Read the model definition and answer for the solid it produces. Units are mm, in the model's axes. Face numbers are marked on the shaded views. Coordinates: 2 decimals unless noted, no trailing zeros. Loops run counter-clockwise (first coordinate to the right, second up) from the corner with the lowest first, then second, coordinate; pieces in that order, holes last. Notation, with made-up numbers: (-16.75, 53.5) -> (20.25, 53.5) arc R25 cw to (20.25, 89.5) -> close; hole circle Ø1 at (32.25, 66). An arc over 180 degrees is marked (long way). Answer as a JSON object with one key per item and string values. Group by question number.
1) Section C-C, the plane y = 28.5 is taken. Give the vertices of the cut face in (x, z).
2) Consider probe 1 along Y at (x, z) = (-7, 5.25); probe 2 along Z at (x, y) = (0, 2); probe 3 along Z at (x, y) = (-52, 55.5). Determine where each line is inside the solid, lowest interval first. Write a range as [from, to].
3) Section A-A, the plane z = -11.5 is taken. Give the vertices of the cut face in (x, y), plus the area to 3 significant figures.
4) Flat-ended cylindrical pins translate along their axes: P1, Ø8.5, axis at x = -14, z = 3, coming from the +Y side; P2, Ø1, axis at x = -11, z = 11, coming from the -Y side; P3, Ø16, axis at y = 40.5, z = 0, coming from the +X side. Find the tip coordinate at first contact, or state that the pin passes through.
5) Section B-B, the plane x = -36 is taken. Give the vertices of the cut face in (y, z).
6) Section D-D, the plane z = 0 is taken. Count the separate pieces of the cut face and the enclosed holes in it, plus the area to 3 significant figures.
7) Determine the mould class of the marked faces 1, 2, 3 and 4 for opening direction Y: released by +Y, released by -Y, zero draft, split by the parting line, or undercut.
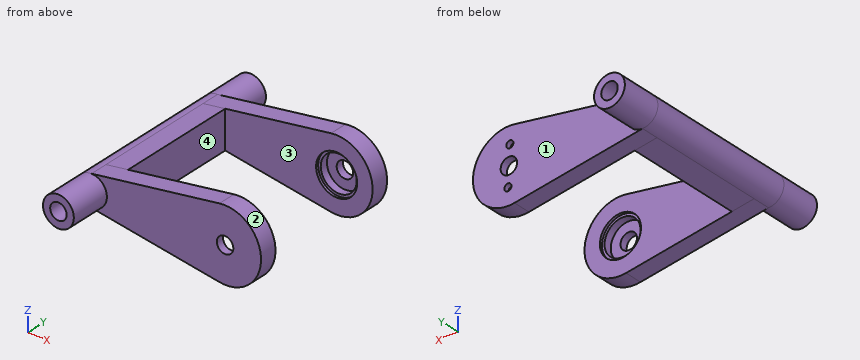
from build123d import *

# Parameters (mm, degrees)
SKETCH1_R               = 3.2
BOSS_EXTRUDE1_DEPTH     = 7
SKETCH2_R               = 3.2
BOSS_EXTRUDE2_DEPTH     = 47
BOSS_EXTRUDE3_OUTLINE_R = 3.2
BOSS_EXTRUDE3_DEPTH     = 7
CUT_EXTRUDE1_DEPTH      = 86.32877599
CUT_EXTRUDE1_DEPTH_BACK = 86.32877599
SKETCH5_R               = 3.2
SKETCH6_R               = 1.395
CUT_EXTRUDE2_DEPTH      = 2
SKETCH7_R               = 7
CUT_EXTRUDE3_DEPTH      = 4
SKETCH8_R               = 8
CUT_EXTRUDE4_DEPTH      = 1
CUT_EXTRUDE5_START      = -4
SKETCH9_R               = 7
CUT_EXTRUDE5_DEPTH      = 4
CUT_EXTRUDE6_START      = -1
SKETCH10_R              = 8
CUT_EXTRUDE6_DEPTH      = 1
SKETCH11_R              = 6
SKETCH11_R_2            = 3.2
BOSS_EXTRUDE4_DEPTH     = 16
BOSS_EXTRUDE5_START     = 16
SKETCH12_R              = 6
SKETCH12_R_2            = 3.2
BOSS_EXTRUDE5_DEPTH     = 16


# Read off the part's stored shape, not the designer's step: Boss-Extrude3
with BuildPart() as part:
    # Sketch1 → Boss-Extrude1 (new body)
    with BuildSketch(Plane(origin=(0, 0, 0), x_dir=(1, 0, 0), z_dir=(0, 1, 0))):
        with BuildLine():
            ThreePointArc((-52, 6), (-58, 0), (-52, -6))
            Line((-52, -6), (-2.173431493, -13.830264184))
            ThreePointArc((-2.173431493, -13.830264184), (14.000000424, -1.65e-07), (-2.173431166, 13.830264236))
            Line((-2.173431166, 13.830264236), (-52, 6))
        make_face()
        with Locations(Location((-52, 0, 0), (0, 0, 270))):
            Circle(SKETCH1_R, mode=Mode.SUBTRACT)
    extrude(amount=BOSS_EXTRUDE1_DEPTH)

    # Sketch2 → Boss-Extrude2 (add)
    # profile 1 of 2: a face of its own
    with BuildSketch(Plane(origin=(0, 7, 0), x_dir=(1, 0, 0), z_dir=(0, 1, 0))):
        with BuildLine():
            ThreePointArc((-46, 0), (-47.757359313, 4.242640687), (-52, 6))
            ThreePointArc((-52, 6), (-58, 0), (-52, -6))
            ThreePointArc((-52, -6), (-47.757359313, -4.242640687), (-46, 0))
        make_face()
        with Locations(Location((-52, 0, 0), (0, 0, 270))):
            Circle(SKETCH2_R, mode=Mode.SUBTRACT)
    # profile 2 of 2: a face of its own
    with BuildSketch(Plane(origin=(0, 7, 0), x_dir=(1, 0, 0), z_dir=(0, 1, 0))):
        with BuildLine():
            Line((-43.357698304, -7.358140997), (-43.357698304, 7.358140997))
            Line((-43.357698304, 7.358140997), (-52, 6))
            ThreePointArc((-52, 6), (-47.757359313, 4.242640687), (-46, 0))
            ThreePointArc((-46, 0), (-47.757359313, -4.242640687), (-52, -6))
            Line((-52, -6), (-43.357698304, -7.358140997))
        make_face()
    extrude(amount=BOSS_EXTRUDE2_DEPTH)

    # Boss-Extrude3 outline → Boss-Extrude3 (add)
    with BuildSketch(Plane(origin=(0, 54, 0), x_dir=(1, 0, 0), z_dir=(0, 1, 0))):
        with BuildLine():
            ThreePointArc((-2.17343128, -13.830264218), (14.000000424, -1.07e-07), (-2.173431068, 13.830264251))
            Line((-2.173431068, 13.830264251), (-52, 6))
            ThreePointArc((-52, 6), (-58, 0), (-52, -6))
            Line((-52, -6), (-2.17343128, -13.830264218))
        make_face()
        with Locations((-52, 0)):
            Circle(BOSS_EXTRUDE3_OUTLINE_R, mode=Mode.SUBTRACT)
    extrude(amount=BOSS_EXTRUDE3_DEPTH)

    # Sketch5 → Cut-Extrude1 (cut, two sides: drawn at the far end of the back side and taken through both)
    with BuildSketch(Plane(origin=(0, 61, 0), x_dir=(1, 0, 0), z_dir=(0, 1, 0)).offset(-CUT_EXTRUDE1_DEPTH_BACK)):
        with Locations(Location((0, 0, 0), (0, 0, 270))):
            Circle(SKETCH5_R)
    extrude(amount=CUT_EXTRUDE1_DEPTH + CUT_EXTRUDE1_DEPTH_BACK, mode=Mode.SUBTRACT)

    # Sketch6 → Cut-Extrude2 (cut)
    with BuildSketch(Plane(origin=(0, 61, 0), x_dir=(1, 0, 0), z_dir=(0, 1, 0))):
        with Locations(Location((-0.370638007, -7.432964974, 0), (0, 0, 270))):
            Circle(SKETCH6_R)
        with Locations(Location((0.370638007, 7.432964974, 0), (0, 0, 270))):
            Circle(SKETCH6_R)
    extrude(amount=-CUT_EXTRUDE2_DEPTH, mode=Mode.SUBTRACT)

    # Sketch7 → Cut-Extrude3 (cut)
    with BuildSketch(Plane.XZ.offset(-54)):
        with Locations(Location((0, 0, 0), (0, 0, 270))):
            Circle(SKETCH7_R)
    extrude(amount=-CUT_EXTRUDE3_DEPTH, mode=Mode.SUBTRACT)

    # Sketch8 → Cut-Extrude4 (cut)
    with BuildSketch(Plane.XZ.offset(-54)):
        with Locations(Location((0, 0, 0), (0, 0, 270))):
            Circle(SKETCH8_R)
    extrude(amount=-CUT_EXTRUDE4_DEPTH, mode=Mode.SUBTRACT)

    # Sketch9 → Cut-Extrude5 (cut)
    with BuildSketch(Plane(origin=(0, 7, 0), x_dir=(1, 0, 0), z_dir=(0, 1, 0)).offset(CUT_EXTRUDE5_START)):
        with Locations(Location((0, 0, 0), (0, 0, 90))):
            Circle(SKETCH9_R)
    extrude(amount=CUT_EXTRUDE5_DEPTH, mode=Mode.SUBTRACT)

    # Sketch10 → Cut-Extrude6 (cut)
    with BuildSketch(Plane(origin=(0, 7, 0), x_dir=(1, 0, 0), z_dir=(0, 1, 0)).offset(CUT_EXTRUDE6_START)):
        with Locations(Location((0, 0, 0), (0, 0, 90))):
            Circle(SKETCH10_R)
    extrude(amount=CUT_EXTRUDE6_DEPTH, mode=Mode.SUBTRACT)

    # Sketch11 → Boss-Extrude4 (add)
    with BuildSketch(Plane(origin=(0, 61, 0), x_dir=(1, 0, 0), z_dir=(0, 1, 0))):
        with Locations(Location((-52, 0, 0), (0, 0, 270))):
            Circle(SKETCH11_R)
        with Locations(Location((-52, 0, 0), (0, 0, 270))):
            Circle(SKETCH11_R_2, mode=Mode.SUBTRACT)
    extrude(amount=BOSS_EXTRUDE4_DEPTH)

    # Sketch12 → Boss-Extrude5 (add)
    with BuildSketch(Plane.XZ.offset(BOSS_EXTRUDE5_START)):
        with Locations(Location((-52, 0, 0), (0, 0, 270))):
            Circle(SKETCH12_R)
        with Locations(Location((-52, 0, 0), (0, 0, 270))):
            Circle(SKETCH12_R_2, mode=Mode.SUBTRACT)
    extrude(amount=-BOSS_EXTRUDE5_DEPTH)


solid = part.part
Determined:
{
 "1": {"outline": "(-52, -6) -> (-43.36, -7.36) -> (-43.36, 7.36) -> (-52, 6) arc R6 ccw to start; hole circle Ø6.4 at (-52, 0)"},
 "2": {"probe 1": "[0, 7], [54, 61]", "probe 2": "[-14, -3.2], [3.2, 14]", "probe 3": "[-6, -3.2], [3.2, 6]"},
 "3": {"outline": "(-17, 0) -> (7.98, 0) -> (7.98, 7) -> (-17, 7) -> close; (-17, 54) -> (7.98, 54) -> (7.98, 61) -> (-17, 61) -> close", "area": "350 mm²"},
 "4": {"P1": "y = 61", "P2": "y = 0", "P3": "x = -43.36"},
 "5": {"outline": "(0, -8.51) -> (7, -8.51) -> (7, 8.51) -> (0, 8.51) -> close; (54, -8.51) -> (61, -8.51) -> (61, 8.51) -> (54, 8.51) -> close"},
 "6": {"separate pieces": "4", "enclosed holes": "0", "area": "1,330 mm²"},
 "7": {"face 1": "released by +Y", "face 2": "zero draft", "face 3": "undercut", "face 4": "undercut"}
}
